from build123d import *

# Parameters (mm, degrees)
SKETCH1_W           = 34
SKETCH1_H           = 30
BOSS_EXTRUDE1_DEPTH = 30
SKETCH2_R           = 5.25
CUT_EXTRUDE1_DEPTH  = 30
SKETCH3_R           = 1.5
CUT_EXTRUDE2_DEPTH  = 15
FILLET1_R           = 1
SKETCH4_R           = 2.15
CUT_EXTRUDE3_DEPTH  = 20


with BuildPart() as part:
    # Sketch1 → Boss-Extrude1 (new body)
    with BuildSketch(Plane.XY):
        with Locations((17, -15)):
            Rectangle(SKETCH1_W, SKETCH1_H)
    extrude(amount=BOSS_EXTRUDE1_DEPTH)

    # Sketch2 → Cut-Extrude1 (cut)
    with BuildSketch(Plane.XY.offset(30)):
        with Locations((17, -15)):
            Circle(SKETCH2_R)
    extrude(amount=-CUT_EXTRUDE1_DEPTH, mode=Mode.SUBTRACT)

    # Sketch3 → Cut-Extrude2 (cut)
    with BuildSketch(Plane.XY.offset(30)):
        with Locations((25, -15)):
            Circle(SKETCH3_R)
        with Locations((17, -7)):
            Circle(SKETCH3_R)
        with Locations((9, -15)):
            Circle(SKETCH3_R)
        with Locations((17, -23)):
            Circle(SKETCH3_R)
    extrude(amount=-CUT_EXTRUDE2_DEPTH, mode=Mode.SUBTRACT)

    # Fillet1
    fillet1_edges = [part.edges().sort_by_distance(p)[0] for p in [
        (34, -15, 30),
        (17, 0, 30),
        (0, -15, 30),
        (17, 0, 0),
        (34, -15, 0),
        (17, -30, 0),
        (0, -15, 0),
        (0, 0, 15),
        (34, 0, 15),
        (34, -30, 15),
        (0, -30, 15),
        (17, -30, 30),
    ]]
    fillet(fillet1_edges, radius=FILLET1_R)

    # Sketch4 → Cut-Extrude3 (cut)
    with BuildSketch(Plane(origin=(0, 0, 0), x_dir=(1, 0, 0), z_dir=(0, 1, 0))):
        with Locations((5, -5)):
            Circle(SKETCH4_R)
        with Locations((29, -5)):
            Circle(SKETCH4_R)
        with Locations((29, -25)):
            Circle(SKETCH4_R)
        with Locations((5, -25)):
            Circle(SKETCH4_R)
    extrude(amount=-CUT_EXTRUDE3_DEPTH, mode=Mode.SUBTRACT)


solid = part.part
Geometry check sheet. Reference: the model listing, model coordinates, mm. A direction names the side the tool comes from. Coordinates: 2 decimals unless noted, no trailing zeros. Order: outer loops, then holes, each group sorted by start corner. A loop starts at its lowest first (then second) coordinate and runs counter-clockwise, first axis right, second up. Notation, with made-up numbers: (23, 23) -> (35, 23) arc R23 cw to (35, 54) -> close; hole circle Ø5 at (-35, -33.75). An arc over 180 degrees is marked (long way). Use a Markdown table: item, result. Add a question column.
1. Cross-section at B-B (z = 14). Enter the section's corners in (x, y).
2. Set-up check for faces 1 (the face through (7.8, -15.9, 22.6)), 2 (the face through (0.285, -0.301, 15.196)), 3 (the face through (29.99, -9.86, 26.91)): record each of +Z, -Z, +X, -X, +Y, -Y from which the full face is reachable in a straight line by a thin tool's end or side.
3. Material ranges on L1, parallel to Y at x = 17, z = 25.5; L2, parallel to Z at x = 5, y = -14.75; L3, parallel to Y at x = 16.5, z = 10.5, recorded low to high.
4. Go/stop test with flat-tipped pins: pin 1 Ø3.5 at (x, z) = (29, 25) entering from +Y; pin 2 Ø1.5 at (x, y) = (8.5, -15) entering from +Z. Record where each tip stops, or that it passes through.
5. Cross-section at C-C (z = 25). Enter the section's corners in (x, y), and give its area (3 significant figures).
6. Mould release check, pull along Y, two halves, no side actions. Record for faces 4 (the face through (15.89, -21.99, 22.6)), 5 (the face through (0, -15, 15)), 6 (the face through (17.224, -29.715, 0.301)): pulls with the +Y half, pulls with the -Y half, needs draft (parallel to the pull), parting line crosses it, or undercut.
7. Cross-section at D-D (x = 5). Enter the section's corners in (y, z).
8. Cross-section at A-A (y = -15). Enter the section's corners in (x, z).
Filled sheet:
| question | item | result |
|---|---|---|
| 1 | outline | (0, -29) arc R1 ccw to (1, -30) -> (33, -30) arc R1 ccw to (34, -29) -> (34, -1) arc R1 ccw to (33, 0) -> (1, 0) arc R1 ccw to (0, -1) -> close; hole circle Ø10.5 at (17, -15) |
| 2 | face 1 | +Z |
| 2 | face 2 | +Z, -Z, -X, +Y |
| 2 | face 3 | +Y |
| 3 | L1 | -30 to -24.5, -21.5 to -20.25, -9.75 to -8.5, -5.5 to 0 |
| 3 | L2 | 0 to 2.85, 7.15 to 22.85, 27.15 to 30 |
| 3 | L3 | -30 to -20.23, -9.77 to 0 |
| 4 | pin 1 | y = -20 |
| 4 | pin 2 | z = 15 |
| 5 | outline | (0, -29) arc R1 ccw to (1, -30) -> (33, -30) arc R1 ccw to (34, -29) -> (34, -1) arc R1 ccw to (33, 0) -> (31.15, 0) -> (31.15, -20) -> (26.85, -20) -> (26.85, 0) -> (7.15, 0) -> (7.15, -20) -> (2.85, -20) -> (2.85, 0) -> (1, 0) arc R1 ccw to (0, -1) -> close; hole circle Ø3 at (9, -15); hole circle Ø10.5 at (17, -15); hole circle Ø3 at (17, -23); hole circle Ø3 at (17, -7); hole circle Ø3 at (25, -15) |
| 5 | area | 732 mm2 |
| 6 | face 4 | undercut |
| 6 | face 5 | needs draft |
| 6 | face 6 | pulls with the -Y half |
| 7 | outline | (-30, 1) arc R1 ccw to (-29, 0) -> (-1, 0) arc R1 ccw to (0, 1) -> (0, 2.85) -> (-20, 2.85) -> (-20, 7.15) -> (0, 7.15) -> (0, 22.85) -> (-20, 22.85) -> (-20, 27.15) -> (0, 27.15) -> (0, 29) arc R1 ccw to (-1, 30) -> (-29, 30) arc R1 ccw to (-30, 29) -> close |
| 8 | outline | (0, 1) arc R1 ccw to (1, 0) -> (11.75, 0) -> (11.75, 30) -> (10.5, 30) -> (10.5, 15) -> (7.5, 15) -> (7.5, 30) -> (1, 30) arc R1 ccw to (0, 29) -> close; (22.25, 0) -> (33, 0) arc R1 ccw to (34, 1) -> (34, 29) arc R1 ccw to (33, 30) -> (26.5, 30) -> (26.5, 15) -> (23.5, 15) -> (23.5, 30) -> (22.25, 30) -> close; hole circle Ø4.3 at (5, 5); hole circle Ø4.3 at (5, 25); hole circle Ø4.3 at (29, 5); hole circle Ø4.3 at (29, 25) |
